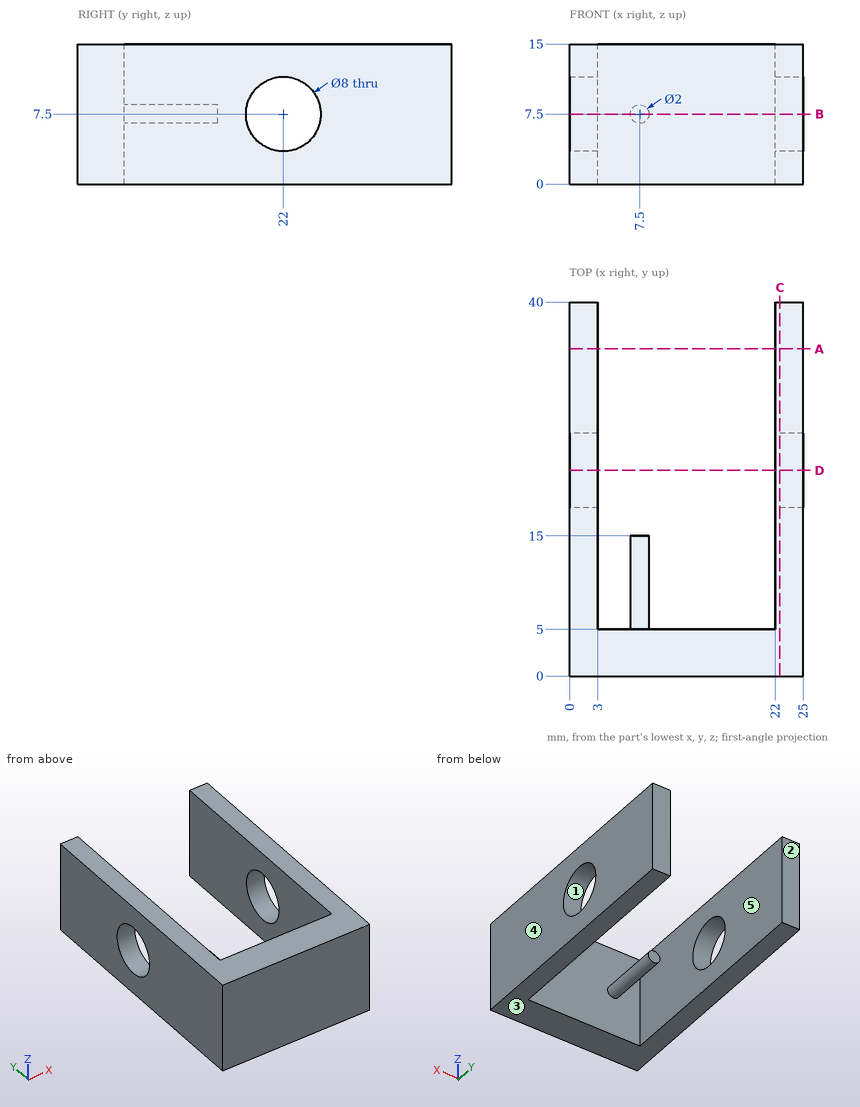
Verification items for this drawing (mm, ordinates from the low corner). A direction names the side the tool comes from. Give positions to 0.01 mm unless a question says otherwise; leave off trailing zeros. Loops run counter-clockwise (first coordinate to the right, second up) from the corner with the lowest first, then second, coordinate; pieces in that order, holes last. Notation, with made-up numbers: M -37.5,2.25 L 15.5,2.25 A17 ccw 15.5,10.25 Z; hole C -27.75,7.5 d8. An arc over 180 degrees is marked long. Answer as a JSON object with one key per item and string values. Group by question number.
Q1. Cross-section at D-D on y = 22. Record the cut outline in (x, z).
Q2. Cross-section at A-A on y = 35. Record the cut outline in (x, z), then the cut area to 3 significant figures.
Q3. Material ranges on line 1 along Y through (x, z) = (22.8, 7.5); line 2 along X through (y, z) = (28, 8); line 3 along Y through (x, z) = (17.75, 14), recorded low to high. Write a range as [from, to].
Q4. Cross-section at C-C on x = 22.5. Record the cut outline in (y, z), then the cut area to 3 significant figures.
Q5. Release check for a two-part mould opening along Z. For the marked faces 1, 2 and 3 record: released by +Z, released by -Z, zero draft, split by the parting line, or undercut.
Q6. Cross-section at B-B on z = 7.5. Record the cut outline in (x, y), then the cut area to 3 significant figures.
Q7. Access from +Z, -Z, +X, -X, +Y, -Y to the whole of each face (thin tool, end or side, straight path). Record for the marked faces 4 and 5.
Q8. Go/stop test with flat-tipped pins: P1, Ø1.5, axis at x = 5, y = 8.5, coming from the -Z side; P2, Ø1.6, axis at x = 7.5, z = 8, coming from the +Y side; P3, Ø6, axis at x = 21.5, z = 11, coming from the +Y side; P4, Ø4.5, axis at x = 17, z = 11, coming from the +Y side. Record where each tip stops, or that it passes through.
Evaluation:
{
 "1": {"outline": "M 0,0 L 3,0 L 3,3.5 L 0,3.5 Z; M 0,11.5 L 3,11.5 L 3,15 L 0,15 Z; M 22,0 L 25,0 L 25,3.5 L 22,3.5 Z; M 22,11.5 L 25,11.5 L 25,15 L 22,15 Z"},
 "2": {"outline": "M 0,0 L 3,0 L 3,15 L 0,15 Z; M 22,0 L 25,0 L 25,15 L 22,15 Z", "area": "90.0 mm2"},
 "3": {"line 1": "y = [0, 18], [26, 40]", "line 2": "x = [0, 3], [22, 25]", "line 3": "y = [0, 5]"},
 "4": {"outline": "M 0,0 L 40,0 L 40,15 L 0,15 Z; hole C 22,7.5 d8", "area": "550 mm2"},
 "5": {"face 1": "undercut", "face 2": "zero draft", "face 3": "released by -Z"},
 "6": {"outline": "M 0,0 L 25,0 L 25,18 L 22,18 L 22,5 L 8.5,5 L 8.5,15 L 6.5,15 L 6.5,5 L 3,5 L 3,18 L 0,18 Z; M 0,26 L 3,26 L 3,40 L 0,40 Z; M 22,26 L 25,26 L 25,40 L 22,40 Z", "area": "307 mm2"},
 "7": {"face 4": "+Z, -Z, +X, +Y, -Y", "face 5": "+Z, -Z, +Y"},
 "8": {"P1": "passes through", "P2": "stops at y = 15", "P3": "stops at y = 40", "P4": "stops at y = 5"}
}
